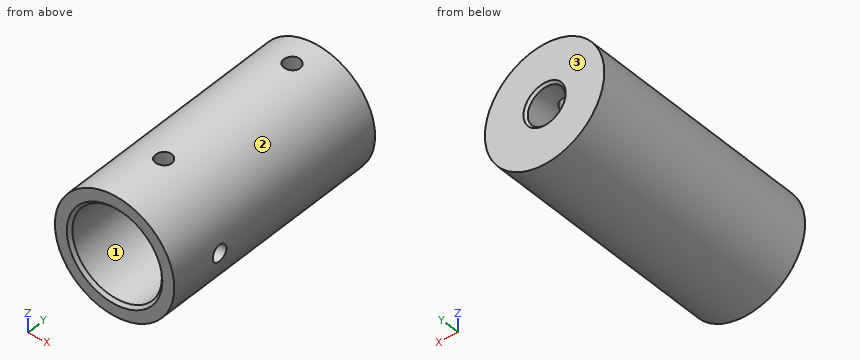
from build123d import *

# Parameters (mm, degrees)
SKETCH1_R                             = 12.7
BOSS_EXTRUDE1_DEPTH                   = 50.8
F_8_0_8_DIAMETER_HOLE1_D              = 8
F_8_0_8_DIAMETER_HOLE1_DEPTH          = 16.51
F_8_0_8_DIAMETER_HOLE1_CSINK_D        = 9
F_8_0_8_DIAMETER_HOLE1_CSINK_ANGLE    = 90
F_8_0_8_DIAMETER_HOLE1_TIP            = 2.403442476
F_8_32_TAPPED_HOLE1_REACH             = 54.894
F_8_32_TAPPED_HOLE1_BORE_R            = 1.7272
F_3_4_0_75_DIAMETER_HOLE1_D           = 19.05
F_3_4_0_75_DIAMETER_HOLE1_DEPTH       = 22.86
F_3_4_0_75_DIAMETER_HOLE1_CSINK_D     = 20.32
F_3_4_0_75_DIAMETER_HOLE1_CSINK_ANGLE = 90
F_3_4_0_75_DIAMETER_HOLE1_TIP         = 5.723197396
TAP_DRILL_FOR_8_32_TAP1_REACH         = 49.733
TAP_DRILL_FOR_8_32_TAP1_BORE_R        = 1.7272
TAP_DRILL_FOR_8_32_TAP2_REACH         = 50.487
TAP_DRILL_FOR_8_32_TAP2_BORE_R        = 1.7272


with BuildPart() as part:
    # Sketch1 → Boss-Extrude1 (new body)
    with BuildSketch(Plane(origin=(0, 0, 0), x_dir=(1, 0, 0), z_dir=(0, 1, 0))):
        with Locations(Location((0, 0, 0), (0, 0, 270))):
            Circle(SKETCH1_R)
    extrude(amount=BOSS_EXTRUDE1_DEPTH)

    # Ø8.0 (8) Diameter Hole1
    with Locations(Plane(origin=(0, 50.8, 0), x_dir=(1, 0, 0), z_dir=(0, 1, 0))):
        with Locations((0, 0)):
            CounterSinkHole(F_8_0_8_DIAMETER_HOLE1_D / 2, F_8_0_8_DIAMETER_HOLE1_CSINK_D / 2, depth=F_8_0_8_DIAMETER_HOLE1_DEPTH, counter_sink_angle=F_8_0_8_DIAMETER_HOLE1_CSINK_ANGLE)
            with Locations((0, 0, -(F_8_0_8_DIAMETER_HOLE1_DEPTH + F_8_0_8_DIAMETER_HOLE1_TIP / 2))):  # 118° drill point
                Cone(0, F_8_0_8_DIAMETER_HOLE1_D / 2, F_8_0_8_DIAMETER_HOLE1_TIP, mode=Mode.SUBTRACT)

    # #8-32 Tapped Hole1 bore (on position points) → #8-32 Tapped Hole1 (cut, up to next)
    with BuildSketch(Plane(origin=(0.258881907, 44.551690017, 12.697361149), x_dir=(0.999792216488, 0, -0.020384402145), z_dir=(0.020384402145, 0, 0.999792216488)), mode=Mode.PRIVATE) as f_8_32_tapped_hole1_sk1:
        Circle(F_8_32_TAPPED_HOLE1_BORE_R)
    f_8_32_tapped_hole1_tool1 = extrude(f_8_32_tapped_hole1_sk1.sketch, amount=-F_8_32_TAPPED_HOLE1_REACH, mode=Mode.PRIVATE) & part.part
    add(f_8_32_tapped_hole1_tool1.solids().sort_by_distance((0.258882, 44.55169, 12.697361))[0], mode=Mode.SUBTRACT)

    # 3/4 (0.75) Diameter Hole1
    with Locations(Plane(origin=(0, 0, 0), x_dir=(-1, 0, 0), z_dir=(0, -1, 0))):
        with Locations((0, 0)):
            CounterSinkHole(F_3_4_0_75_DIAMETER_HOLE1_D / 2, F_3_4_0_75_DIAMETER_HOLE1_CSINK_D / 2, depth=F_3_4_0_75_DIAMETER_HOLE1_DEPTH, counter_sink_angle=F_3_4_0_75_DIAMETER_HOLE1_CSINK_ANGLE)
            with Locations((0, 0, -(F_3_4_0_75_DIAMETER_HOLE1_DEPTH + F_3_4_0_75_DIAMETER_HOLE1_TIP / 2))):  # 118° drill point
                Cone(0, F_3_4_0_75_DIAMETER_HOLE1_D / 2, F_3_4_0_75_DIAMETER_HOLE1_TIP, mode=Mode.SUBTRACT)

    # Tap Drill for #8-32 Tap1 bore (on position points) → Tap Drill for #8-32 Tap1 (cut, up to next)
    with BuildSketch(Plane(origin=(-0.035098468, 12.444517797, 12.6999515), x_dir=(0.999996181087, 0, 0.002763658925), z_dir=(-0.002763658925, 0, 0.999996181087)), mode=Mode.PRIVATE) as tap_drill_for_8_32_tap1_sk1:
        Circle(TAP_DRILL_FOR_8_32_TAP1_BORE_R)
    tap_drill_for_8_32_tap1_tool1 = extrude(tap_drill_for_8_32_tap1_sk1.sketch, amount=-TAP_DRILL_FOR_8_32_TAP1_REACH, mode=Mode.PRIVATE) & part.part
    add(tap_drill_for_8_32_tap1_tool1.solids().sort_by_distance((-0.035098, 12.444518, 12.699951))[0], mode=Mode.SUBTRACT)

    # Tap Drill for #8-32 Tap2 bore (on position points) → Tap Drill for #8-32 Tap2 (cut, up to next)
    with BuildSketch(Plane(origin=(12.7, 11.499385571, 0), x_dir=(0, 0, 1), z_dir=(1, 0, 0)), mode=Mode.PRIVATE) as tap_drill_for_8_32_tap2_sk1:
        Circle(TAP_DRILL_FOR_8_32_TAP2_BORE_R)
    tap_drill_for_8_32_tap2_tool1 = extrude(tap_drill_for_8_32_tap2_sk1.sketch, amount=-TAP_DRILL_FOR_8_32_TAP2_REACH, mode=Mode.PRIVATE) & part.part
    add(tap_drill_for_8_32_tap2_tool1.solids().sort_by_distance((12.7, 11.499386, 0))[0], mode=Mode.SUBTRACT)


solid = part.part
The model under review builds one solid part; all positions refer to its coordinate system, in mm. Face numbers are marked on the shaded views. Round coordinates to 2 decimals unless told otherwise and drop trailing zeros. Write each loop counter-clockwise with the first axis right and the second up, starting at its lowest first coordinate (ties: lowest second). Pieces come first, ordered by that corner, then holes. Notation, with made-up numbers: M -29,66 L 23,66 A21 cw 23,100 Z; hole C -29,65.25 d4. An arc over 180 degrees is marked long. Answer as CSV lines item,"result". Start each with the question number.
Q1. Consider section B-B, the plane x = -0.5. State how many separate pieces and enclosed holes the cut face has, then the cut area to 3 significant figures.
Q2. Wall thickness on line 1 along Z through (x, y) = (-0.25, 36); line 2 along Z through (x, y) = (1.5, 36); line 3 along X through (y, z) = (25, -1): over which ranges is each line inside the solid? List them lowest first.
Q3. The part is to be moulded in two halves that separate along X. For the marked faces 1, 2 and 3, say which applies: +X half, -X half, draft (parallel to the pull), parting line (faces both ways), or undercut.
Q4. Consider section A-A, the plane y = 18. Give the boundary of the cut face in (x, z) (3 decimals).
Q5. Consider section C-C, the plane x = -10.75. Give the boundary of the cut face in (y, z).
Q6. Clearance check with flat-ended pins moving along their axes: P1, Ø1.5, axis at y = 13.5, z = -5.5, coming from the -X side; P2, Ø1.5, axis at x = -7.5, y = 5.5, coming from the +Z side; P3, Ø8, axis at x = -8.5, y = 7, coming from the +Z side. State where each tip first meets the part, or that it passes through.
Result set:
1,separate pieces,"3"
1,enclosed holes,"0"
1,area,"621 mm²"
2,line 1,"z = -12.7 to -3.99, 3.99 to 12.7"
2,line 2,"z = -12.61 to -3.71, 3.71 to 12.61"
2,line 3,"x = -12.66 to -5.88, 5.88 to 12.66"
3,face 1,"undercut"
3,face 2,"parting line"
3,face 3,"draft"
4,outline,"C 0,0 d25.4; hole C 0,0 d19.05"
5,outline,"M 0,-6.76 L 50.8,-6.76 L 50.8,6.76 L 0,6.76 Z"
6,P1,"stops at x = -11.78"
6,P2,"stops at z = 10.76"
6,P3,"stops at z = 11.88"
